from build123d import *

# Parameters (mm, degrees)
CUT_EXTRUDE1_DEPTH                        = 3
F_5_0MM_DOWEL_HOLE1_D                     = 5
F_5_0MM_DOWEL_HOLE1_DEPTH                 = 10
F_5_0MM_DOWEL_HOLE1_CSINK_D               = 5.05
F_5_0MM_DOWEL_HOLE1_CSINK_ANGLE           = 90
F_5_0MM_DOWEL_HOLE1_TIP                   = 1.502151548
F_5_0MM_DOWEL_HOLE1_ON_FACE_2_D           = 5
F_5_0MM_DOWEL_HOLE1_ON_FACE_2_DEPTH       = 10
F_5_0MM_DOWEL_HOLE1_ON_FACE_2_CSINK_D     = 5.05
F_5_0MM_DOWEL_HOLE1_ON_FACE_2_CSINK_ANGLE = 90
F_5_0MM_DOWEL_HOLE1_ON_FACE_2_TIP         = 1.502151548


with BuildPart() as part:
    # Sketch1 → Revolve1 (revolve)
    with BuildSketch(Plane.XY):
        Polygon((0, 0), (0, 10), (50, 10), (50, 12.5), (60, 12.5), (60, 10), (110, 10), (110, 0), align=None)
    revolve(axis=Axis((110, 0, 0), (-1, 0, 0)))

    # Sketch2 → Cut-Extrude1 (cut)
    with BuildSketch(Plane(origin=(0, 10, 0), x_dir=(1, 0, 0), z_dir=(0, 1, 0))):
        with BuildLine():
            Line((47, -3), (28, -3))
            ThreePointArc((28, -3), (25, 0), (28, 3))
            Line((28, 3), (47, 3))
            ThreePointArc((47, 3), (50, 0), (47, -3))
        make_face()
        with BuildLine():
            Line((63, 3), (82, 3))
            ThreePointArc((82, 3), (85, 0), (82, -3))
            Line((82, -3), (63, -3))
            ThreePointArc((63, -3), (60, 0), (63, 3))
        make_face()
    extrude(amount=-CUT_EXTRUDE1_DEPTH, mode=Mode.SUBTRACT)

    # Ø5.0mm Dowel Hole1
    with Locations(Plane.YZ.offset(110)):
        with Locations((0, 0)):
            CounterSinkHole(F_5_0MM_DOWEL_HOLE1_D / 2, F_5_0MM_DOWEL_HOLE1_CSINK_D / 2, depth=F_5_0MM_DOWEL_HOLE1_DEPTH, counter_sink_angle=F_5_0MM_DOWEL_HOLE1_CSINK_ANGLE)
            with Locations((0, 0, -(F_5_0MM_DOWEL_HOLE1_DEPTH + F_5_0MM_DOWEL_HOLE1_TIP / 2))):  # 118° drill point
                Cone(0, F_5_0MM_DOWEL_HOLE1_D / 2, F_5_0MM_DOWEL_HOLE1_TIP, mode=Mode.SUBTRACT)

    # Ø5.0mm Dowel Hole1 on face 2
    with Locations(Plane(origin=(0, 0, 0), x_dir=(0, 0, -1), z_dir=(-1, 0, 0))):
        with Locations((0, 0)):
            CounterSinkHole(F_5_0MM_DOWEL_HOLE1_ON_FACE_2_D / 2, F_5_0MM_DOWEL_HOLE1_ON_FACE_2_CSINK_D / 2, depth=F_5_0MM_DOWEL_HOLE1_ON_FACE_2_DEPTH, counter_sink_angle=F_5_0MM_DOWEL_HOLE1_ON_FACE_2_CSINK_ANGLE)
            with Locations((0, 0, -(F_5_0MM_DOWEL_HOLE1_ON_FACE_2_DEPTH + F_5_0MM_DOWEL_HOLE1_ON_FACE_2_TIP / 2))):  # 118° drill point
                Cone(0, F_5_0MM_DOWEL_HOLE1_ON_FACE_2_D / 2, F_5_0MM_DOWEL_HOLE1_ON_FACE_2_TIP, mode=Mode.SUBTRACT)


solid = part.part
The listing builds one solid part. Answer for the finished solid, in the listing's coordinates (mm). A direction names the side the tool comes from. Give positions to 0.01 mm unless a question says otherwise; leave off trailing zeros. Write each loop counter-clockwise with the first axis right and the second up, starting at its lowest first coordinate (ties: lowest second). Pieces come first, ordered by that corner, then holes.
1) Given P1, Ø2, axis at x = 39, y = 8.5, coming from the -Z side; P2, Ø3, axis at x = 72, y = 8.5, coming from the +Z side; P3, Ø4, axis at y = 0, z = 0, coming from the -X side, each flat-ended and moving along its own axis, determine where each tip first touches the part or whether it passes through.
2) Section C-C (z = 5) is taken. Write down the section's boundary in (x, y), and give its area (3 significant figures).
3) For a pull along Z with two mould halves and no side action, classify faces 1 (the face through (25.35, -2.17, 9.76)), 2 (the face through (5.08, 2.44, -0.54)), 3 (the face through (60, -0.1, -10.2)) as pulls with the +Z half, pulls with the -Z half, needs draft (parallel to the pull), parting line crosses it, or undercut.
4) Section B-B (x = 18.5) is taken. Write down the section's boundary in (y, z).
5) Section A-A (y = -3.5) is taken. Write down the section's boundary in (x, z), and give its area (3 significant figures).
6) Find the intervals of material crossed by L1, parallel to Y at x = 2.75, z = 0; L2, parallel to X at y = 0, z = 10.5, in increasing order.
7) Section D-D (x = 61.5) is taken. Write down the section's boundary in (y, z).
8) A tool of negligible diameter and unlimited length cuts with its end or side. For faces 4 (the face through (73, 7, 0)), 5 (the face through (55.07, 11.923, -3.755)), 6 (the face through (50, 0.1, -10.2)), 7 (the face through (85.35, -2.17, 9.76)), from which of +Z, -Z, +X, -X, +Y, -Y can it reach the whole face along a straight path? Write none if from no direction.
Response:
1. P1: stops at z = -6.61
1. P2: stops at z = 7.14
1. P3: stops at x = 10.3
2. outline: (0, -8.66) - (50, -8.66) - (50, -11.46) - (60, -11.46) - (60, -8.66) - (110, -8.66) - (110, 8.66) - (60, 8.66) - (60, 11.46) - (50, 11.46) - (50, 8.66) - (0, 8.66) - close
2. area: 1,960 mm2
3. face 1: parting line crosses it
3. face 2: undercut
3. face 3: needs draft
4. outline: circle Ø20 at (0, 0)
5. outline: (0, -9.37) - (50, -9.37) - (50, -12) - (60, -12) - (60, -9.37) - (110, -9.37) - (110, 9.37) - (60, 9.37) - (60, 12) - (50, 12) - (50, 9.37) - (0, 9.37) - close
5. area: 2,110 mm2
6. L1: y = -10 to -2.5, 2.5 to 10
6. L2: x = 50 to 60
7. outline: (7, -2.6) - (7, 2.6) - (9.66, 2.6) arc R10 ccw (long way) to (9.66, -2.6) - close
8. face 4: +Y
8. face 5: +X, -X
8. face 6: -X
8. face 7: +X
